Can you work these out from the drawing? Everything is in mm from the part's minimum corner. A direction names the side the tool comes from. Coordinates: 2 decimals unless noted, no trailing zeros. Order: outer loops, then holes, each group sorted by start corner. A loop starts at its lowest first (then second) coordinate and runs counter-clockwise, first axis right, second up. Notation, with made-up numbers: (64.25, 65) - (118.25, 65) arc R18 cw to (118.25, 84) - close; hole circle Ø2 at (64.5, 58). An arc over 180 degrees is marked (long way). Use CSV: the item, a comma, the result in double quotes. Start each with the question number.
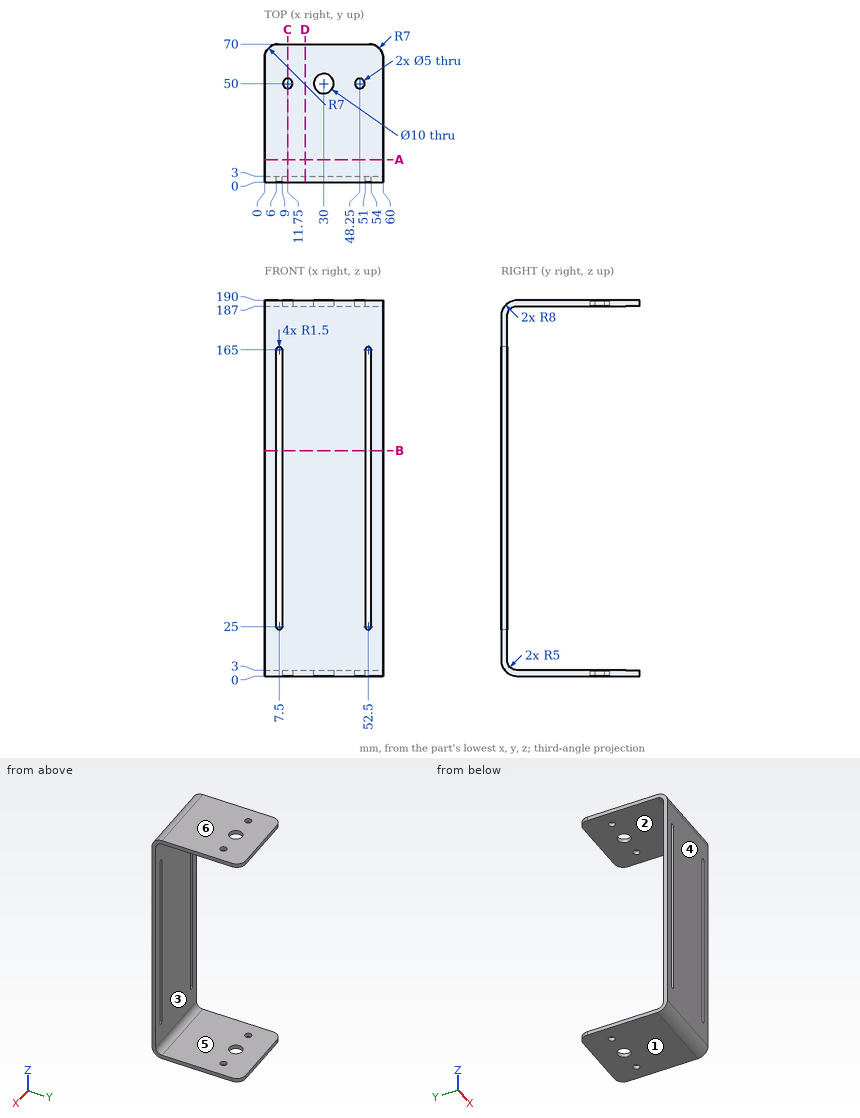
Item 1: For pin 1 Ø6 at (x, y) = (30, 50) entering from +Z; pin 2 Ø8 at (x, z) = (40.5, 158.5) entering from +Y; pin 3 Ø6.5 at (x, y) = (48.25, 50) entering from +Z, each with a flat end and sliding along its axis, tell me the tip position at first contact or that it passes through.
Item 2: Suppose I cut it at B-B on z = 114. Write out the boundary of the cut face in (x, y).
Item 3: For the marked faces 5 and 6, which set-ups out of +Z, -Z, +X, -X, +Y, -Y let a thin tool reach every point of the face, with its end or its side?
Item 4: Suppose I cut it at A-A on y = 11.5. Write out the boundary of the cut face in (x, z).
Item 5: Please list where these lines run through material, in increasing order: line 1 along Z through (x, y) = (6.5, 62.5); line 2 along Z through (x, y) = (54.5, 4.5); line 3 along Y through (x, z) = (50, 134). Write a range as from..to.
Item 6: We'd pull the mould along Z, two halves only. Please class the marked faces 1, 2, 3 and 4: released by +Z, released by -Z, zero draft, split by the parting line, or undercut.
Item 7: Suppose I cut it at C-C on x = 11.75. Write out the boundary of the cut face in (y, z).
Item 8: Suppose I cut it at D-D on x = 20.5. Write out the boundary of the cut face in (y, z).
Here are the results:
1,pin 1,"through"
1,pin 2,"y = 3"
1,pin 3,"z = 190"
2,outline,"(0, 0) - (6, 0) - (6, 3) - (0, 3) - close; (9, 0) - (51, 0) - (51, 3) - (9, 3) - close; (54, 0) - (60, 0) - (60, 3) - (54, 3) - close"
3,face 5,"+X, -X, +Y"
3,face 6,"+Z, +X, -X, +Y, -Y"
4,outline,"(0, 0) - (60, 0) - (60, 3) - (0, 3) - close; (0, 187) - (60, 187) - (60, 190) - (0, 190) - close"
5,line 1,"0..3, 187..190"
5,line 2,"0.81..4.43, 185.57..189.19"
5,line 3,"0..3"
6,face 1,"released by -Z"
6,face 2,"undercut"
6,face 3,"undercut"
6,face 4,"zero draft"
7,outline,"(0, 8) arc R8 ccw to (8, 0) - (47.5, 0) - (47.5, 3) - (8, 3) arc R5 cw to (3, 8) - (3, 182) arc R5 cw to (8, 187) - (47.5, 187) - (47.5, 190) - (8, 190) arc R8 ccw to (0, 182) - close; (52.5, 0) - (70, 0) - (70, 3) - (52.5, 3) - close; (52.5, 187) - (70, 187) - (70, 190) - (52.5, 190) - close"
8,outline,"(0, 8) arc R8 ccw to (8, 0) - (70, 0) - (70, 3) - (8, 3) arc R5 cw to (3, 8) - (3, 182) arc R5 cw to (8, 187) - (70, 187) - (70, 190) - (8, 190) arc R8 ccw to (0, 182) - close"
